Source: three-view drawing plus pictorial views. Frame: mm from the lowest corner of the part. A direction names the side the tool comes from. Round coordinates to 2 decimals unless told otherwise and drop trailing zeros. Loops run counter-clockwise (first coordinate to the right, second up) from the corner with the lowest first, then second, coordinate; pieces in that order, holes last. Notation, with made-up numbers: (42.5, 87.25) -> (49.5, 87.25) arc R5 cw to (49.5, 93.25) -> close; hole circle Ø11 at (50, -11.75). An arc over 180 degrees is marked (long way). Return JSON: item names as keys, results as strings. Group by question number.
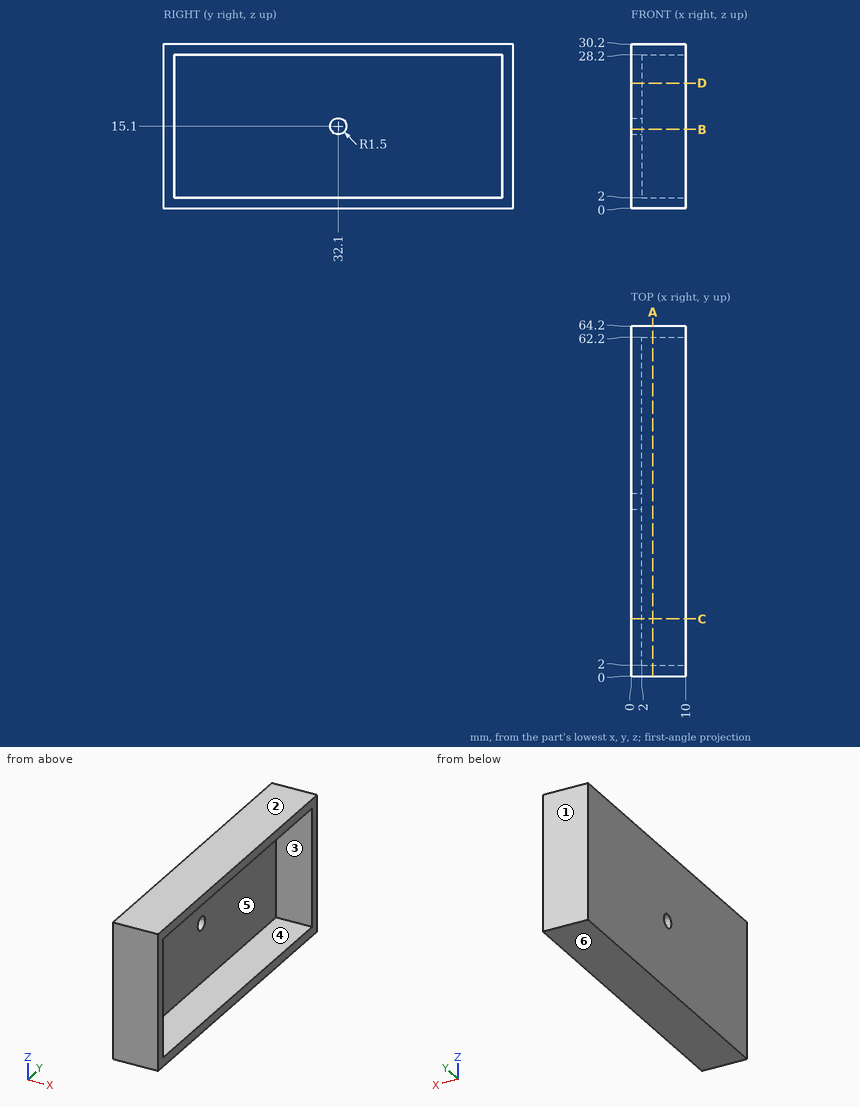
(1) Pin query (flat end, axial travel): pin 1 (13 mm diameter, centred on y = 28.5, z = 20.5, fed in from +X). Return the tip coordinate at first contact, or that it passes through.
(2) Set-up query: the marked faces 5 and 6. Return all of +Z, -Z, +X, -X, +Y, -Y with unobstructed straight access to the full face (end or side cutting, diameter ignored); none if empty.
(3) Cut plane D-D (z = 23). Return loops of the section in (x, y), and give its area (3 significant figures).
(4) Ray query, line 1 (Y direction, x = 8.25, z = 26); line 2 (Z direction, x = 5.75, y = 59.5); line 3 (X direction, y = 53, z = 19). Return the intervals inside material, ascending.
(5) Cut plane C-C (y = 10.5). Return loops of the section in (x, z), and give its area (3 significant figures).
(6) Mould query, pull axis Z, two halves, no side actions, for the marked faces 1, 2, 3 and 4. Classes: released by +Z, released by -Z, zero draft, split by the parting line, or undercut.
(7) Cut plane A-A (x = 4). Return loops of the section in (y, z).
(8) Cut plane B-B (z = 14.5). Return loops of the section in (x, y).
Answers follow:
{
 "1": {"pin 1": "x = 2"},
 "2": {"face 5": "+X", "face 6": "-Z, +X, -X, +Y, -Y"},
 "3": {"outline": "(0, 0) -> (10, 0) -> (10, 2) -> (2, 2) -> (2, 62.2) -> (10, 62.2) -> (10, 64.2) -> (0, 64.2) -> close", "area": "160 mm^2"},
 "4": {"line 1": "0 to 2, 62.2 to 64.2", "line 2": "0 to 2, 28.2 to 30.2", "line 3": "0 to 2"},
 "5": {"outline": "(0, 0) -> (10, 0) -> (10, 2) -> (2, 2) -> (2, 28.2) -> (10, 28.2) -> (10, 30.2) -> (0, 30.2) -> close", "area": "92.4 mm^2"},
 "6": {"face 1": "zero draft", "face 2": "released by +Z", "face 3": "undercut", "face 4": "undercut"},
 "7": {"outline": "(0, 0) -> (64.2, 0) -> (64.2, 30.2) -> (0, 30.2) -> close; hole (2, 2) -> (62.2, 2) -> (62.2, 28.2) -> (2, 28.2) -> close"},
 "8": {"outline": "(0, 0) -> (10, 0) -> (10, 2) -> (2, 2) -> (2, 30.73) -> (0, 30.73) -> close; (0, 33.47) -> (2, 33.47) -> (2, 62.2) -> (10, 62.2) -> (10, 64.2) -> (0, 64.2) -> close"}
}
